The listing builds one solid part. Answer for the finished solid, in the listing's coordinates (mm). A direction names the side the tool comes from. Round coordinates to 2 decimals unless told otherwise and drop trailing zeros. Write each loop counter-clockwise with the first axis right and the second up, starting at its lowest first coordinate (ties: lowest second). Pieces come first, ordered by that corner, then holes. Notation, with made-up numbers: M -4,83.5 L 7,83.5 A27 ccw 7,113.5 Z; hole C -38.75,-16 d7. An arc over 180 degrees is marked long. One line per item, written item: value. Start each with the question number.
(1) Section A-A (y = -111.5) is taken. Determine the outline of the cut face in (x, z) (3 decimals), plus the area to 3 significant figures.
(2) Section D-D (x = 85) is taken. Determine the outline of the cut face in (y, z).
(3) Section B-B (z = 0.9) is taken. Determine the outline of the cut face in (x, y) (3 decimals), plus the area to 3 significant figures.
(4) Section C-C (x = 60.25) is taken. Determine the outline of the cut face in (y, z), plus the area to 3 significant figures.
(5) Consider probe 1 along Y at (x, z) = (73, 1.1); probe 2 along X at (y, z) = (-99, 0.2) (3 decimals); probe 3 along Y at (x, z) = (75.25, 1.05). Determine where each line is inside the solid, lowest interval first.
(6) For faces 4 (the flat face through (69.065, -102, 1)), 5 (the flat face through (77, -127, 1)), determine the directions among +Z, -Z, +X, -X, +Y, -Y from which every point of the face is accessible in a straight line to the end or side of a thin tool.
(7) Given P1, Ø2.5, axis at x = 74.94, y = -115, coming from the +Z side, flat-ended and moving along its own axis, determine where the tip first touches the part or whether it passes through.
(8) For a pull along Y with two mould halves and no side action, classify faces 1 (the flat face through (72, -116.5, 1)), 2 (the flat face through (87, -92, 1)), 3 (the cylindrical face through (85.289, -78.804, 0.76)) as released by +Y, released by -Y, zero draft, split by the parting line, or undercut.
Autodesk Inventor part; units mm, degrees
ref_plane "YZ Plane" through (0, 0, 0) normal (1, 0, 0) x (0, 1, 0)
ref_plane "XZ Plane" through (0, 0, 0) normal (0, 1, 0) x (-1, 0, 0)
ref_plane "XY Plane" through (0, 0, 0) normal (0, 0, 1) x (1, 0, 0)
sketch "Sketch2" plane through (0, 0, 0) normal (0, 0, 1) x (1, 0, 0)
  line L0 (0, 0) -> (144, 0) construction
  line L1 (144, 0) -> (144, -204) construction
  line L2 (144, -204) -> (0, -204) construction
  line L3 (0, -204) -> (0, 0) construction
  circle A0 centre (135, -27) radius 3 construction
  circle A1 centre (122, -9) radius 3 construction
  circle A2 centre (135, -177) radius 3 construction
  circle A3 centre (122, -195) radius 3 construction
  circle A4 centre (22, -195) radius 3 construction
  circle A5 centre (9, -177) radius 3 construction
  circle A6 centre (9, -27) radius 3 construction
  circle A7 centre (22, -9) radius 3 construction
  line L4 (12, -12) -> (132, -12) construction
  line L5 (132, -12) -> (132, -192) construction
  line L6 (132, -192) -> (12, -192) construction
  line L7 (12, -192) -> (12, -12) construction
  circle A8 centre (22, -9) radius 2.925
  circle A9 centre (9, -27) radius 2.925
  circle A10 centre (122, -9) radius 2.925
  circle A11 centre (135, -27) radius 2.925
  circle A12 centre (135, -177) radius 2.925
  circle A13 centre (122, -195) radius 2.925
  circle A14 centre (22, -195) radius 2.925
  circle A15 centre (9, -177) radius 2.925
  line L8 (122, -9) -> (135, -9) construction
  line L9 (135, -9) -> (135, -27) construction
  line L10 (126, -27) -> (126, -18)
  line L11 (126, -18) -> (122, -18)
  line L12 (144, -27) -> (144, 0)
  line L13 (144, 0) -> (122, 0)
  line L14 (122, -195) -> (135, -195) construction
  line L15 (135, -195) -> (135, -177) construction
  line L16 (126, -177) -> (126, -186)
  line L17 (126, -186) -> (122, -186)
  line L18 (144, -177) -> (144, -204)
  line L19 (144, -204) -> (122, -204)
  line L20 (126, -27) -> (126, -177)
  line L21 (144, -177) -> (144, -27)
  line L22 (122, -9) -> (113, -9) construction
  line L23 (122, 0) -> (113, 0)
  line L24 (122, -18) -> (113, -18)
  line L25 (113, -18) -> (113, 0)
  line L26 (122, -195) -> (113, -195) construction
  line L27 (122, -204) -> (113, -204)
  line L28 (122, -186) -> (113, -186)
  line L29 (113, -186) -> (113, -204)
  line L30 (75.025, -87) -> (68.975, -87) construction
  line L31 (68.975, -87) -> (68.975, -117) construction
  line L32 (68.975, -117) -> (75.025, -117) construction
  line L33 (75.025, -117) -> (75.025, -87) construction
  line L34 (74.935, -87.5) -> (73.6121, -87.5)
  line L35 (69.065, -87.5) -> (69.065, -91)
  line L36 (69.065, -116.5) -> (70.3879, -116.5)
  line L37 (74.935, -116.5) -> (74.935, -113)
  arc A16 (73.6121, -116.5) -> (74.935, -113) centre (74.935, -115) ccw
  arc A17 (69.065, -113) -> (70.3879, -116.5) centre (69.065, -115) ccw
  arc A18 (74.935, -91) -> (73.6121, -87.5) centre (74.935, -89) ccw
  arc A19 (70.3879, -87.5) -> (69.065, -91) centre (69.065, -89) ccw
  line L38 (69.065, -91) -> (69.065, -113)
  line L39 (70.3879, -87.5) -> (69.065, -87.5)
  line L40 (73.6121, -87.5) -> (70.3879, -87.5)
  line L41 (74.935, -91) -> (74.935, -87.5)
  line L42 (74.935, -113) -> (74.935, -91)
  line L43 (70.3879, -116.5) -> (73.6121, -116.5)
  line L44 (73.6121, -116.5) -> (74.935, -116.5)
  line L45 (69.065, -113) -> (69.065, -116.5)
  arc A20 (69.065, -91) -> (70.3879, -87.5) centre (69.065, -89) ccw
  arc A21 (73.6121, -87.5) -> (74.935, -91) centre (74.935, -89) ccw
  arc A22 (74.935, -113) -> (73.6121, -116.5) centre (74.935, -115) ccw
  arc A23 (70.3879, -116.5) -> (69.065, -113) centre (69.065, -115) ccw
  line L46 (57, -127) -> (87, -127)
  line L47 (87, -127) -> (87, -77)
  line L48 (87, -77) -> (57, -77)
  line L49 (57, -77) -> (57, -127)
  point P0 (132, -102)
  point P1 (144, -102)
  point P2 (72, -12)
  point P3 (72, 0)
  point P4 (72, -87)
  point P5 (75.025, -102)
  point P6 (74.935, -102)
  point P7 (72, -87.5)
  point P8 (74.935, -102)
  point P9 (72, -87.5)
  point P10 (72, -77)
  point P11 (87, -102)
  dimension "d0" = 144
  dimension "d1" = 204
  dimension "d2" = 6
  dimension "d3" = 6
  dimension "d4" = 6
  dimension "d5" = 6
  dimension "d6" = 6
  dimension "d7" = 6
  dimension "d8" = 6
  dimension "d9" = 6
  dimension "d10" = 120
  dimension "d11" = 180
  dimension "d12" = 15
  dimension "d13" = 10
  dimension "d14" = 10
  dimension "d15" = 15
  dimension "d16" = 15
  dimension "d17" = 10
  dimension "d18" = 10
  dimension "d19" = 15
  dimension "d20" = 0.075
  dimension "d21" = 0.075
  dimension "d22" = 0.075
  dimension "d23" = 0.075
  dimension "d24" = 0.075
  dimension "d25" = 0.075
  dimension "d26" = 0.075
  dimension "d27" = 0.075
  dimension "d28" = 9
  dimension "d29" = 9
  dimension "d30" = 9
  dimension "d31" = 9
  dimension "d32" = 9
  dimension "d33" = 9
  dimension "d34" = 6.05
  dimension "d35" = 30
  dimension "d36" = 29
  dimension "d37" = 5.87
  dimension "d38" = 4
  dimension "d39" = 1.5
  dimension "d40" = 4
  dimension "d41" = 1.5
  dimension "d42" = 1.5
  dimension "d43" = 1.5
  dimension "d44" = 4
  dimension "d45" = 4
  dimension "d54" = 30
  dimension "d55" = 50
extrude "Extrusion1" add sketch "Sketch2" along normal blind 1.5 contours L49 L48 L47 L46
sketch "Sketch3" plane through (0, 0, 1.5) normal (0, 0, 1) x (1, 0, 0)
  line L0 (87, -77) -> (57, -77) construction
  line L1 (72, -77) -> (72, -78.5) construction
  line L2 (57, -127) -> (87, -127) construction
  line L3 (72, -127) -> (72, -125.5) construction
  line L4 (57, -77) -> (57, -127) construction
  line L5 (57, -102) -> (58.5, -102) construction
  line L6 (87, -127) -> (87, -77) construction
  line L7 (87, -102) -> (85.5, -102) construction
  line L8 (72, -78.5) -> (72.866, -77)
  line L9 (72, -78.5) -> (73.7321, -78.5) construction
  line L10 (72, -78.5) -> (71.134, -77)
  line L11 (71.134, -77) -> (72.866, -77)
  line L12 (72, -125.5) -> (72.866, -127)
  line L13 (72, -125.5) -> (71.134, -127)
  line L14 (72.866, -127) -> (71.134, -127)
  line L15 (58.5, -102) -> (57, -101.134)
  line L16 (57, -102.866) -> (58.5, -102)
  line L17 (57, -101.134) -> (57, -102.866)
  line L18 (85.5, -102) -> (87, -101.134)
  line L19 (85.5, -102) -> (87, -102.866)
  line L20 (87, -101.134) -> (87, -102.866)
  point P0 (0, 0)
  dimension "d59" = 1.5
  dimension "d60" = 1.5
  dimension "d61" = 1.5
  dimension "d62" = 1.5
  dimension "d63" = 60
  dimension "d64" = 60
  dimension "d65" = 60
  dimension "d66" = 60
  dimension "d67" = 60
extrude "Extrusion2" cut sketch "Sketch3" against normal blind 1.5
fillet "Fillet1" radius 6 4 edges at (57, -127, 0.75) (87, -127, 0.75) (87, -77, 0.75) (57, -77, 0.75)
equation "\"d0\" = d46"
equation "\"d1\" = d47"
equation "\"d2\" = d48"
equation "\"d3\" = d48"
equation "\"d4\" = d48"
equation "\"d5\" = d48"
equation "\"d6\" = d48"
equation "\"d7\" = d48"
equation "\"d8\" = d48"
equation "\"d9\" = d48"
equation "\"d10\" = d49"
equation "\"d11\" = d50"
equation "\"d12\" = d51"
equation "\"d13\" = d52"
equation "\"d14\" = d52"
equation "\"d15\" = d51"
equation "\"d16\" = d51"
equation "\"d17\" = d52"
equation "\"d18\" = d52"
equation "\"d19\" = d51"
equation "\"d20\" = d53"
equation "\"d21\" = d53"
equation "\"d22\" = d53"
equation "\"d23\" = d53"
equation "\"d24\" = d53"
equation "\"d25\" = d53"
equation "\"d26\" = d53"
equation "\"d27\" = d53"
equation "\"d28\" = 1.5 * d48"
equation "\"d29\" = 1.5 * d48"
equation "\"d30\" = 1.5 * d48"
equation "\"d31\" = 1.5 * d48"
equation "\"d32\" = 1.5 * d48"
equation "\"d33\" = 1.5 * d48"
equation "\"d40\" = d38"
equation "\"d41\" = d39"
equation "\"d42\" = d39"
equation "\"d43\" = d42"
equation "\"d44\" = d38"
equation "\"d45\" = d38"
equation "\"d60\" = d59"
equation "\"d61\" = d59"
equation "\"d62\" = d59"
properties part number "pcb-holder"
Recorded:
1. outline: M 57,0 L 69.065,0 L 69.065,1.5 L 57,1.5 Z; M 74.935,0 L 87,0 L 87,1.5 L 74.935,1.5 Z
1. area: 36.2 mm2
2. outline: M -125.47,0 L -78.53,0 L -78.53,1.5 L -125.47,1.5 Z
3. outline: M 57,-121 A6 ccw 63,-127 L 71.134,-127 L 72,-125.5 L 72.866,-127 L 81,-127 A6 ccw 87,-121 L 87,-102.866 L 85.5,-102 L 87,-101.134 L 87,-83 A6 ccw 81,-77 L 72.866,-77 L 72,-78.5 L 71.134,-77 L 63,-77 A6 ccw 57,-83 L 57,-101.134 L 58.5,-102 L 57,-102.866 Z; hole M 69.065,-113 A2 ccw long 70.388,-116.5 L 73.612,-116.5 A2 ccw long 74.935,-113 L 74.935,-91 A2 ccw long 73.612,-87.5 L 70.388,-87.5 A2 ccw long 69.065,-91 Z
3. area: 1,270 mm2
4. outline: M -126.33,0 L -77.67,0 L -77.67,1.5 L -126.33,1.5 Z
4. area: 73.0 mm2
5. probe 1: y = -127 to -116.5, -87.5 to -77
5. probe 2: x = 57 to 69.065, 74.935 to 87
5. probe 3: y = -127 to -116.98, -113.02 to -90.98, -87.02 to -77
6. face 4: +Z, -Z
6. face 5: +Z, -Z, +X, -X, -Y
7. P1: passes through
8. face 1: undercut
8. face 2: zero draft
8. face 3: released by +Y
